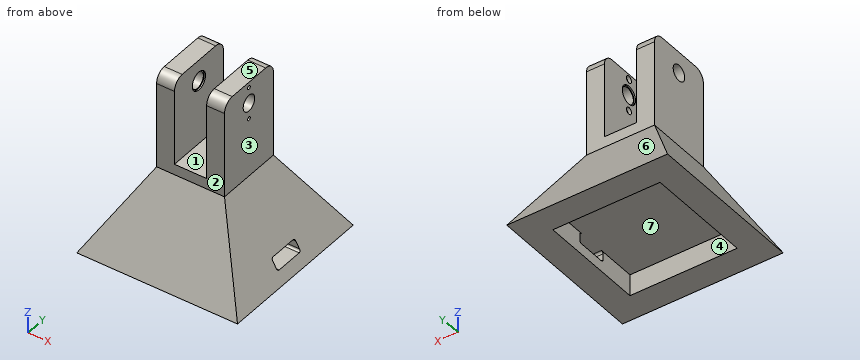
```python
from build123d import *

# Parameters (mm, degrees)
SKETCH2_W           = 150
SKETCH2_H           = 150
BOSS_EXTRUDE1_DEPTH = 75
BOSS_EXTRUDE1_TAPER = 30
SKETCH3_W           = 63.397459622
SKETCH3_H           = 63.397459622
BOSS_EXTRUDE2_DEPTH = 90
SKETCH4_W           = 30
SKETCH4_H           = 63.397459622
CUT_EXTRUDE1_DEPTH  = 80
FILLET1_R           = 10
CUT_EXTRUDE2_REACH  = 249.204
SKETCH5_R           = 7.5
SKETCH6_W           = 100
SKETCH6_H           = 100
CUT_EXTRUDE3_DEPTH  = 20
SKETCH7_W           = 10
SKETCH7_H           = 30
CUT_EXTRUDE4_DEPTH  = 256.636460623
FILLET2_R           = 2
SKETCH8_R           = 1.75
CUT_EXTRUDE5_DEPTH  = 16.698729811
CUT_EXTRUDE6_START  = -3
SKETCH9_R           = 3.25
SKETCH9_R_2         = 1.75
CUT_EXTRUDE6_DEPTH  = 3
SKETCH10_R          = 8.6
CUT_EXTRUDE7_DEPTH  = 1.25


with BuildPart() as part:
    # Sketch2 → Boss-Extrude1 (new body)
    with BuildSketch(Plane.XY):
        with Locations((75, 75)):
            Rectangle(SKETCH2_W, SKETCH2_H)
    extrude(amount=BOSS_EXTRUDE1_DEPTH, taper=BOSS_EXTRUDE1_TAPER)

    # Sketch3 → Boss-Extrude2 (add)
    with BuildSketch(Plane.XY.offset(75)):
        with Locations((75, 75)):
            Rectangle(SKETCH3_W, SKETCH3_H)
    extrude(amount=BOSS_EXTRUDE2_DEPTH)

    # Sketch4 → Cut-Extrude1 (cut)
    with BuildSketch(Plane.XY.offset(165)):
        with Locations((75, 75)):
            Rectangle(SKETCH4_W, SKETCH4_H)
    extrude(amount=-CUT_EXTRUDE1_DEPTH, mode=Mode.SUBTRACT)

    # Fillet1
    fillet1_edges = [part.edges().sort_by_distance(p)[0] for p in [
        (98.349364905, 106.698729811, 165),
        (51.650635095, 43.301270189, 165),
        (51.650635095, 106.698729811, 165),
        (98.349364905, 43.301270189, 165),
    ]]
    fillet(fillet1_edges, radius=FILLET1_R)

    # Cut-Extrude2: up to this face of the body (flat: up to its plane)
    cut_extrude2_end = Plane(part.part.faces().sort_by_distance((106.698729811, 75, 119.675861825))[0])
    # Sketch5 → Cut-Extrude2 (cut, up to the picked face)
    with BuildSketch(Plane.ZY.offset(-43.301270189), mode=Mode.PRIVATE) as cut_extrude2_sk1:
        with Locations((145, 75)):
            Circle(SKETCH5_R)
    cut_extrude2_tool1 = split(extrude(cut_extrude2_sk1.sketch, amount=-CUT_EXTRUDE2_REACH, mode=Mode.PRIVATE), bisect_by=cut_extrude2_end, keep=Keep.BOTH, mode=Mode.PRIVATE)
    add(cut_extrude2_tool1.solids().sort_by(Axis((43.30127, 75, 145), (1, 0, 0)))[0], mode=Mode.SUBTRACT)

    # Sketch6 → Cut-Extrude3 (cut)
    with BuildSketch(Plane(origin=(0, 0, 0), x_dir=(-1, 0, 0), z_dir=(0, 0, -1))):
        with Locations((-75, 75)):
            Rectangle(SKETCH6_W, SKETCH6_H)
    extrude(amount=-CUT_EXTRUDE3_DEPTH, mode=Mode.SUBTRACT)

    # Sketch7 → Cut-Extrude4 (cut, through all)
    with BuildSketch(Plane.ZY.offset(-125)):
        with Locations((15, 75)):
            Rectangle(SKETCH7_W, SKETCH7_H)
    extrude(amount=-CUT_EXTRUDE4_DEPTH, mode=Mode.SUBTRACT)

    # Fillet2
    fillet2_edges = [part.edges().sort_by_distance(p)[0] for p in [
        (131.726497308, 90, 20),
        (131.726497308, 60, 20),
        (134.613248654, 60, 10),
        (134.613248654, 90, 10),
    ]]
    fillet(fillet2_edges, radius=FILLET2_R)

    # Sketch8 → Cut-Extrude5 (cut)
    with BuildSketch(Plane(origin=(106.698729811, 0, 0), x_dir=(0, 0, -1), z_dir=(1, 0, 0))):
        with Locations((-160, 75)):
            Circle(SKETCH8_R)
        with Locations((-130, 75)):
            Circle(SKETCH8_R)
    extrude(amount=-CUT_EXTRUDE5_DEPTH, mode=Mode.SUBTRACT)

    # Sketch9 → Cut-Extrude6 (cut)
    # profile 1 of 2: a face of its own
    with BuildSketch(Plane.ZY.offset(-90).offset(CUT_EXTRUDE6_START)):
        with Locations(Location((160, 75, 0), (0, 0, 270))):
            Circle(SKETCH9_R)
        with Locations(Location((160, 75, 0), (0, 0, 180))):
            Circle(SKETCH9_R_2, mode=Mode.SUBTRACT)
    # profile 2 of 2: a face of its own
    with BuildSketch(Plane.ZY.offset(-90).offset(CUT_EXTRUDE6_START)):
        with Locations(Location((130, 75, 0), (0, 0, 270))):
            Circle(SKETCH9_R)
        with Locations(Location((130, 75, 0), (0, 0, 180))):
            Circle(SKETCH9_R_2, mode=Mode.SUBTRACT)
    extrude(amount=CUT_EXTRUDE6_DEPTH, mode=Mode.SUBTRACT)

    # Sketch10 → Cut-Extrude7 (cut)
    with BuildSketch(Plane(origin=(60, 0, 0), x_dir=(0, 0, -1), z_dir=(1, 0, 0))):
        with Locations(Location((-145, 75, 0), (0, 0, 90))):
            Circle(SKETCH10_R)
    cut_extrude7 = extrude(amount=-CUT_EXTRUDE7_DEPTH, mode=Mode.SUBTRACT)

    # Mirror1: Cut-Extrude7 across plane
    add(cut_extrude7.mirror(Plane(origin=(75, 0, 0), x_dir=(0, 0, 1), z_dir=(1, 0, 0))), mode=Mode.SUBTRACT)


solid = part.part
```
The listing builds one solid part. Answer for the finished solid, in the listing's coordinates (mm). Face numbers are marked on the shaded views. A direction names the side the tool comes from. Give positions to 0.01 mm unless a question says otherwise; leave off trailing zeros. Order: outer loops, then holes, each group sorted by start corner. A loop starts at its lowest first (then second) coordinate and runs counter-clockwise, first axis right, second up.
1) For the marked faces 1, 2, 3 and 4, determine the directions among +Z, -Z, +X, -X, +Y, -Y from which every point of the face is accessible in a straight line to the end or side of a thin tool.
Reported:
face 1: +Z, +Y, -Y
face 2: +Z, +X, -X, -Y
face 3: +Z, +X, +Y, -Y
face 4: -Z
2) Find section A-A on z = 145. Write down the section's boundary in (x, y).
Reported:
outline: (43.3, 43.3) - (60, 43.3) - (60, 66.4) - (58.75, 66.4) - (58.75, 67.5) - (43.3, 67.5) - close; (43.3, 82.5) - (58.75, 82.5) - (58.75, 83.6) - (60, 83.6) - (60, 106.7) - (43.3, 106.7) - close; (90, 43.3) - (106.7, 43.3) - (106.7, 67.5) - (91.25, 67.5) - (91.25, 66.4) - (90, 66.4) - close; (90, 83.6) - (91.25, 83.6) - (91.25, 82.5) - (106.7, 82.5) - (106.7, 106.7) - (90, 106.7) - close
3) Consider line 1 along Y through (x, z) = (100, 130); line 2 along X through (y, z) = (55.5, 131); line 3 along Z through (x, y) = (59, 75). Determine where each line is inside the solid, lowest interval first.
Reported:
line 1: y = 43.3 to 73.25, 76.75 to 106.7
line 2: x = 43.3 to 60, 90 to 106.7
line 3: z = 20 to 136.4, 153.6 to 165
4) Find section C-C on z = 116.5. Write down the section's boundary in (x, y).
Reported:
outline: (43.3, 43.3) - (60, 43.3) - (60, 106.7) - (43.3, 106.7) - close; (90, 43.3) - (106.7, 43.3) - (106.7, 106.7) - (90, 106.7) - close
5) Given P1, Ø22.5, axis at y = 75, z = 145, coming from the +X side; P2, Ø5, axis at y = 76, z = 160.5, coming from the -X side; P3, Ø10, axis at y = 60.5, z = 12.5, coming from the -X side; P4, Ø5, axis at y = 71, z = 144, coming from the +X side, each flat-ended and moving along its own axis, determine where each tip first touches the part or whether it passes through.
Reported:
P1: stops at x = 106.7
P2: stops at x = 43.3
P3: stops at x = 4.33
P4: passes through
6) Find section B-B on x = 98. Write down the section's boundary in (y, z), then the cut area to 3 significant figures.
Reported:
outline: (0, 0) - (25, 0) - (25, 20) - (125, 20) - (125, 0) - (150, 0) - (106.7, 75) - (106.7, 155) arc R10 ccw to (96.7, 165) - (53.3, 165) arc R10 ccw to (43.3, 155) - (43.3, 75) - close; hole circle Ø15 at (75, 145); hole circle Ø3.5 at (75, 130); hole circle Ø3.5 at (75, 160)
area: 11,500 mm2
7) Find section D-D on x = 36.5. Write down the section's boundary in (y, z).
Reported:
outline: (0, 0) - (25, 0) - (25, 20) - (125, 20) - (125, 0) - (150, 0) - (113.5, 63.22) - (36.5, 63.22) - close
8) Determine the mould class of the marked faces 5, 6 and 7 for opening direction Y: pulls with the +Y half, pulls with the -Y half, needs draft (parallel to the pull), parting line crosses it, or undercut.
Reported:
face 5: needs draft
face 6: pulls with the +Y half
face 7: undercut
